Input: part model. Units: mm. Frame: model coordinates. A direction names the side the tool comes from. Round coordinates to 2 decimals unless told otherwise and drop trailing zeros. Order: outer loops, then holes, each group sorted by start corner. A loop starts at its lowest first (then second) coordinate and runs counter-clockwise, first axis right, second up. Notation, with made-up numbers: (-8.75, -34) -> (25.25, -34) arc R12 cw to (25.25, -18) -> close; hole circle Ø10 at (28.25, -15). An arc over 180 degrees is marked (long way). Use a Markdown table: item, result.
from build123d import *

# Parameters (mm, degrees)
F0_W     = 236.2
F0_H     = 154.8
F0_W_2   = 160
F0_H_2   = 104
F1_DEPTH = 5
F2_R     = 17
F3_R     = 3.25
F4_DEPTH = 2.5
F5_SIZE2 = 4.99999
F5_SIZE  = 1.624588
F7_DEPTH = 1.5


# Not quite as in the source:
# - a fillet or chamfer is up to 0.001 mm smaller than in the source, because OpenCascade refuses the exact size


with BuildPart() as f1:
    # F0 (on Front) → F1 (new body)
    with BuildSketch(Plane.XZ):
        Rectangle(F0_W, F0_H)
        Rectangle(F0_W_2, F0_H_2, mode=Mode.SUBTRACT)
    extrude(amount=F1_DEPTH)

    # F2
    f2_edges = [f1.edges().sort_by_distance(p)[0] for p in [
        (-118.1, -2.5, 77.4),
        (118.1, -2.5, 77.4),
        (-118.1, -2.5, -77.4),
        (118.1, -2.5, -77.4),
    ]]
    fillet(f2_edges, radius=F2_R)

    # F3 (on face) → F4 (cut)
    with BuildSketch(Plane(origin=(0, 0, 0), x_dir=(-1, 0, 0), z_dir=(0, 1, 0))):
        with Locations((-79.25, 66.42428)):
            Circle(F3_R)
        with Locations((-79.25, -66.42428)):
            Circle(F3_R)
        with Locations((79.25, 66.42428)):
            Circle(F3_R)
        with Locations((79.25, -66.42428)):
            Circle(F3_R)
    extrude(amount=-F4_DEPTH, mode=Mode.SUBTRACT)

    # F5 (size 1.6245984812 and 5 in the source; OpenCascade refuses exactly that, so slightly less here)
    f5_edges = [f1.edges().sort_by_distance(p)[0] for p in [
        (-80, -5, 0),
        (0, -5, 52),
        (80, -5, 0),
        (0, -5, -52),
    ]]
    f5_side = f1.faces().sort_by_distance((0, -5, 74.575934))[0]
    chamfer(f5_edges, length=F5_SIZE, length2=F5_SIZE2, reference=f5_side)

    # F6 (on face) → F7 (cut)
    with BuildSketch(Plane.XZ.offset(5)):
        with BuildLine():
            Line((0, -70.9037960887), (0, -68.7403732376))
            Line((0, -68.7403732376), (-3.125376912, -68.8479899255))
            ThreePointArc((-3.125376912, -68.8479899255), (-3.7805726372, -68.5735525412), (-3.998605605, -67.897491197))
            Line((-3.998605605, -67.897491197), (-3.0892937711, -60.2992490469))
            ThreePointArc((-3.0892937711, -60.2992490469), (-3.1618997395, -60.0916194181), (-3.3704565536, -60.021721316))
            Line((-3.3704565536, -60.021721316), (-5.3485393199, -60.2845971301))
            ThreePointArc((-5.3485393199, -60.2845971301), (-5.5237209211, -60.3724524554), (-5.6072790976, -60.5497239497))
            Line((-5.6072790976, -60.5497239497), (-6.4865739197, -68.6796104252))
            ThreePointArc((-6.4865739197, -68.6796104252), (-5.9450748854, -70.3262933271), (-4.3499759171, -71.004854352))
            Line((-4.3499759171, -71.004854352), (0, -70.9037960887))
        make_face()
        with BuildLine():
            Line((1.2918589674, -60.2652083751), (0, -60.3707235945))
            Line((0, -60.3707235945), (0, -66.8485857862))
            Line((0, -66.8485857862), (3.4268085146, -66.6858144104))
            Line((3.4268085146, -66.6858144104), (3.0311800837, -70.6349397286))
            ThreePointArc((3.0311800837, -70.6349397286), (3.0818813973, -70.7890639463), (3.2301839467, -70.8548761904))
            Line((3.2301839467, -70.8548761904), (5.0478271442, -70.8548761904))
            ThreePointArc((5.0478271442, -70.8548761904), (5.1809587177, -70.8041276029), (5.2465278981, -70.6776360316))
            Line((5.2465278981, -70.6776360316), (6.4378099563, -60.2773594464))
            ThreePointArc((6.4378099563, -60.2773594464), (6.3777706296, -60.1104711604), (6.2086864979, -60.0569269995))
            Line((6.2086864979, -60.0569269995), (4.2790884308, -60.3539008339))
            ThreePointArc((4.2790884308, -60.3539008339), (4.1073828743, -60.4436163854), (4.0263119894, -60.6195686231))
            Line((4.0263119894, -60.6195686231), (3.6252996651, -64.4996576011))
            Line((3.6252996651, -64.4996576011), (1.0174442614, -64.6235291889))
            Line((1.0174442614, -64.6235291889), (1.506754727, -60.4880446531))
            ThreePointArc((1.506754727, -60.4880446531), (1.4521032332, -60.3257114675), (1.2918589674, -60.2652083751))
        make_face()
        with BuildLine():
            Line((0, -66.8485857862), (0, -60.3707235945))
            Line((0, -60.3707235945), (-0.7053982188, -60.4283384346))
            ThreePointArc((-0.7053982188, -60.4283384346), (-0.8907958695, -60.512923053), (-0.9793808578, -60.6964429332))
            Line((-0.9793808578, -60.6964429332), (-1.552537239, -66.2315062229))
            ThreePointArc((-1.552537239, -66.2315062229), (-1.3916459971, -66.7055871007), (-0.9272608372, -66.892630127))
            Line((-0.9272608372, -66.892630127), (0, -66.8485857862))
        make_face()
        with BuildLine():
            Line((0.7437746725, -68.7147627052), (0, -68.7403732376))
            Line((0, -68.7403732376), (0, -70.9037960887))
            Line((0, -70.9037960887), (0.4531291197, -70.8932690322))
            ThreePointArc((0.4531291197, -70.8932690322), (0.6476972416, -70.8155735275), (0.7439755724, -70.6294987347))
            Line((0.7439755724, -70.6294987347), (0.9491999954, -68.9387434307))
            ThreePointArc((0.9491999954, -68.9387434307), (0.8980521088, -68.7794601123), (0.7437746725, -68.7147627052))
        make_face()
    extrude(amount=-F7_DEPTH, mode=Mode.SUBTRACT)


solid = f1.part
1) Pin query (flat end, axial travel): pin 1 Ø6 at (x, z) = (79.25, 66.42) entering from +Y; pin 2 Ø5 at (x, z) = (78, -66) entering from +Y. Return the tip coordinate at first contact, or that it passes through.
Results found:
| item | result |
|---|---|
| pin 1 | stops at y = -2.5 |
| pin 2 | stops at y = 0 |
2) Pull-direction query (X, two-part tool) for faces 4 (the flat face through (-118.1, -2, -1)), 5 (the flat face through (118.1, -2, -1)), 6 (the flat face through (-79, -2.5, 66)); classes: +X half, -X half, draft (parallel to the pull), parting line (faces both ways), or undercut.
Results found:
| item | result |
|---|---|
| face 4 | -X half |
| face 5 | +X half |
| face 6 | undercut |
3) Cut plane C-C on y = -1.5. Return loops of the section in (x, z), and give its area (3 significant figures).
Results found:
| item | result |
|---|---|
| outline | (-118.1, -60.4) arc R17 ccw to (-101.1, -77.4) -> (101.1, -77.4) arc R17 ccw to (118.1, -60.4) -> (118.1, 60.4) arc R17 ccw to (101.1, 77.4) -> (-101.1, 77.4) arc R17 ccw to (-118.1, 60.4) -> close; hole circle Ø6.5 at (-79.25, -66.42); hole circle Ø6.5 at (-79.25, 66.42); hole (-80.49, -52.49) -> (80.49, -52.49) -> (80.49, 52.49) -> (-80.49, 52.49) -> close; hole circle Ø6.5 at (79.25, -66.42); hole circle Ø6.5 at (79.25, 66.42) |
| area | 19,300 mm² |
4) Line query: L1, parallel to Z at x = -3, y = -0.3; L2, parallel to Z at x = 26, y = -3.5; L3, parallel to X at y = -1.7, z = 15.5. Output: solid intervals per line, ascending. Write a range as [from, to].
Results found:
| item | result |
|---|---|
| L1 | z = [-77.4, -52.1], [52.1, 77.4] |
| L2 | z = [-77.4, -53.14], [53.14, 77.4] |
| L3 | x = [-118.1, -80.55], [80.55, 118.1] |
5) Set-up query: faces 1 (the flat face through (-2, 0, 53)), 2 (the flat face through (80.801, -2.465, -0.751)), 3 (the cylindrical face through (81.83, -1.23, 64.45)). Return all of +Z, -Z, +X, -X, +Y, -Y with unobstructed straight access to the full face (end or side cutting, diameter ignored); none if empty.
Results found:
| item | result |
|---|---|
| face 1 | +Z, -Z, +X, -X, +Y |
| face 2 | -Y |
| face 3 | +Y |
